from build123d import *

# Parameters (mm, degrees)
F1_DEPTH = 25.4
F2_DEPTH = 25.4


with BuildPart() as f1:
    # F0 (on Top) → F1 (new body)
    with BuildSketch(Plane.XY):
        with BuildLine():
            Line((33.487893, 38.1), (-42.712107, 38.1))
            Line((-42.712107, 38.1), (-42.712107, 0))
            Line((-42.712107, 0), (-18.949738, 0))
            ThreePointArc((-18.949738, 0), (-2.707106, 22.487095), (13.535526, 0))
            Line((13.535526, 0), (33.487893, 0))
            Line((33.487893, 0), (33.487893, 38.1))
        make_face()
        with BuildLine():
            ThreePointArc((13.535526, 0), (-2.707106, 22.487095), (-18.949738, 0))
            Line((-18.949738, 0), (13.535526, 0))
        make_face()
    extrude(amount=F1_DEPTH)

    # F0 (on Top) → F2 (cut)
    with BuildSketch(Plane.XY):
        with BuildLine():
            ThreePointArc((13.535526, 0), (-2.707106, 22.487095), (-18.949738, 0))
            Line((-18.949738, 0), (13.535526, 0))
        make_face()
    extrude(amount=F2_DEPTH, mode=Mode.SUBTRACT)


solid = f1.part
Source: CAD feature listing. Evaluate the final solid. Frame: model axes, mm. Round coordinates to 2 decimals unless told otherwise and drop trailing zeros. Write each loop counter-clockwise with the first axis right and the second up, starting at its lowest first coordinate (ties: lowest second). Pieces come first, ordered by that corner, then holes. Notation, with made-up numbers: M -38.75,64.25 L 13.25,64.25 A24 ccw 13.25,81.25 Z; hole C -6,25 d11. An arc over 180 degrees is marked long. One line per item, written item: value. Start each with the question number.
Item 1: Mould query, pull axis Y, two halves, no side actions, for faces 1 (the cylindrical face through (-2.25, 22.48, 12.52)), 2 (the flat face through (-4, 38.1, 13)), 3 (the flat face through (23, 0, 13)), 4 (the flat face through (-42.712, 19, 13)). Classes: pulls with the +Y half, pulls with the -Y half, needs draft (parallel to the pull), parting line crosses it, or undercut.
Item 2: Ray query, L1, parallel to X at y = 5, z = 4.5; L2, parallel to Y at x = -3, z = 10; L3, parallel to X at y = 16, z = 4.75. Return the intervals inside material, ascending. Write a range as from..to.
Item 3: Section query A-A (y = 17). Return the cut outline in (x, z).
Item 4: Section query C-C (y = 7). Return the cut outline in (x, z).
Item 5: Pin query (flat end, axial travel): pin 1 (8 mm diameter, centred on x = -11, z = 12, fed in from -Y). Return the tip coordinate at first contact, or that it passes through.
Item 6: Section query D-D (x = -17.5). Return the cut outline in (y, z), plus the area to 3 significant figures.
Item 7: Section query B-B (z = 19.5). Return the cut outline in (x, y).
Result set:
1. face 1: undercut
1. face 2: pulls with the +Y half
1. face 3: pulls with the -Y half
1. face 4: needs draft
2. L1: x = -42.71..-19.81, 14.4..33.49
2. L2: y = 22.48..38.1
2. L3: x = -42.71..-16.12, 10.71..33.49
3. outline: M -42.71,0 L -15.26,0 L -15.26,25.4 L -42.71,25.4 Z; M 9.85,0 L 33.49,0 L 33.49,25.4 L 9.85,25.4 Z
4. outline: M -42.71,0 L -19.74,0 L -19.74,25.4 L -42.71,25.4 Z; M 14.33,0 L 33.49,0 L 33.49,25.4 L 14.33,25.4 Z
5. pin 1: stops at y = 17.28
6. outline: M 13.97,0 L 38.1,0 L 38.1,25.4 L 13.97,25.4 Z
6. area: 613 mm²
7. outline: M -42.71,0 L -18.95,0 A17.11 cw long 13.54,0 L 33.49,0 L 33.49,38.1 L -42.71,38.1 Z
